Design review of the part built by this model. Coordinates are the model's own, in mm. A direction names the side the tool comes from. Coordinates: 2 decimals unless noted, no trailing zeros. Loops run counter-clockwise (first coordinate to the right, second up) from the corner with the lowest first, then second, coordinate; pieces in that order, holes last.
from build123d import *

# Parameters (mm, degrees)
SKETCH1_R           = 5.55625
BOSS_EXTRUDE1_DEPTH = 1.5875
SKETCH2_R           = 3.96875
SKETCH2_R_2         = 2.38125
EXTRUDE_THIN1_DEPTH = 11.1125
FILLET1_R           = 0.254


with BuildPart() as part:
    # Sketch1 → Boss-Extrude1 (new body)
    with BuildSketch(Plane(origin=(0, 0, 0), x_dir=(1, 0, 0), z_dir=(0, 1, 0))):
        with Locations(Location((0, 0, 0), (0, 0, 270))):
            Circle(SKETCH1_R)
    extrude(amount=BOSS_EXTRUDE1_DEPTH)

    # Sketch2 → Extrude-Thin1 (add)
    with BuildSketch(Plane(origin=(0, 1.5875, 0), x_dir=(1, 0, 0), z_dir=(0, 1, 0))):
        Circle(SKETCH2_R)
        Circle(SKETCH2_R_2, mode=Mode.SUBTRACT)
    extrude(amount=EXTRUDE_THIN1_DEPTH)

    # Fillet1
    fillet1_edges = [part.edges().sort_by_distance(p)[0] for p in [
        (0, 0, -5.55625),
    ]]
    fillet(fillet1_edges, radius=FILLET1_R)


solid = part.part
Q1. The part is to be moulded in two halves that separate along Z. For faces 1 (the flat face through (0, 1.588, 0)), 2 (the cylindrical face through (4.685, 0.911, 2.987)), 3 (the flat face through (1, 1.588, -4)), say which applies: pulls with the +Z half, pulls with the -Z half, needs draft (parallel to the pull), parting line crosses it, or undercut.
Q2. Machinability: for faces 4 (the cylindrical face through (-0.86, 7.066, 3.874)), 5 (the flat face through (2, 12.7, 2)), which of the approach directions +Z, -Z, +X, -X, +Y, -Y give a long, thin tool a straight path to every point of the face, cutting with its end or side? Answer none if there is none.
Q3. Take a section at B-B, the plane y = 9.75. Write out the cut boundary in (x, z).
Q4. For line 1 (Z direction, x = 0, y = 9); line 2 (Y direction, x = 0, z = -5), list the stretches that pass through material, from the lowest coordinate up.
Q5. Take a section at C-C, the plane z = 0. Write out the cut boundary in (x, y), then the cut area to 3 significant figures.
Q6. Clearance check with flat-ended pins moving along their axes: pin 1 Ø1.5 at (x, z) = (3.5, 4) entering from +Y; pin 2 Ø2 at (y, z) = (8.5, 0) entering from -X; pin 3 Ø5 at (x, y) = (2, 7) entering from +Z. State where each tip first meets the part, or that it passes through.
Q7. Take a section at A-A, the plane x = 0. Write out the cut boundary in (y, z), then the cut area to 3 significant figures.
Entries:
1. face 1: undercut
1. face 2: parting line crosses it
1. face 3: needs draft
2. face 4: +Y
2. face 5: +Z, -Z, +X, -X, +Y
3. outline: circle Ø7.94 at (0, 0); hole circle Ø4.76 at (0, 0)
4. line 1: z = -3.97 to -2.38, 2.38 to 3.97
4. line 2: y = 0 to 1.59
5. outline: (-5.56, 0.25) arc R0.25 ccw to (-5.3, 0) - (5.3, 0) arc R0.25 ccw to (5.56, 0.25) - (5.56, 1.59) - (3.97, 1.59) - (3.97, 12.7) - (2.38, 12.7) - (2.38, 1.59) - (-2.38, 1.59) - (-2.38, 12.7) - (-3.97, 12.7) - (-3.97, 1.59) - (-5.56, 1.59) - close
5. area: 52.9 mm2
6. pin 1: stops at y = 1.59
6. pin 2: stops at x = -3.97
6. pin 3: stops at z = 3.97
7. outline: (0, -5.3) arc R0.25 ccw to (0.25, -5.56) - (1.59, -5.56) - (1.59, -3.97) - (12.7, -3.97) - (12.7, -2.38) - (1.59, -2.38) - (1.59, 2.38) - (12.7, 2.38) - (12.7, 3.97) - (1.59, 3.97) - (1.59, 5.56) - (0.25, 5.56) arc R0.25 ccw to (0, 5.3) - close
7. area: 52.9 mm2
